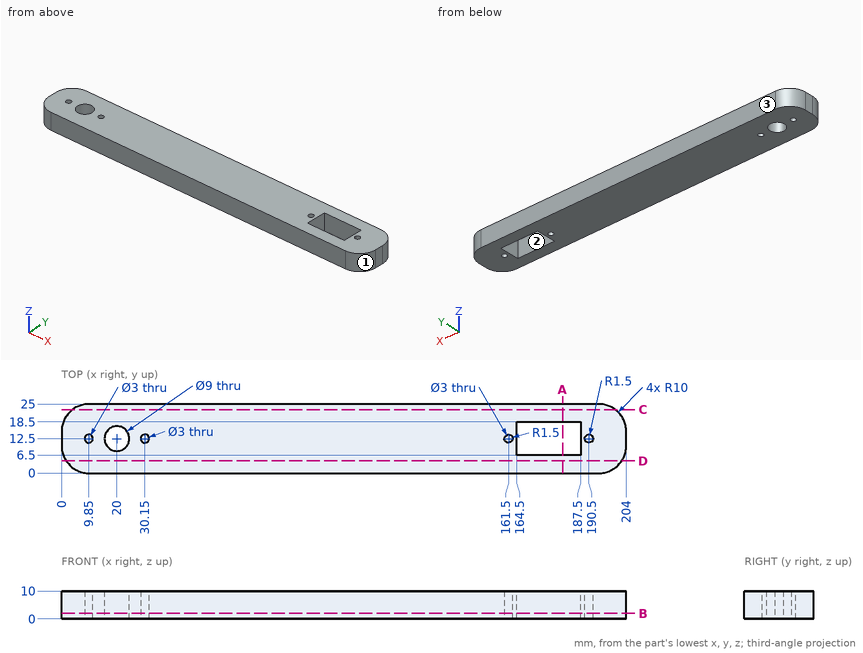
Can you work these out from the drawing? Everything is in mm from the part's minimum corner. Round coordinates to 2 decimals unless told otherwise and drop trailing zeros. Loops run counter-clockwise (first coordinate to the right, second up) from the corner with the lowest first, then second, coordinate; pieces in that order, holes last. Notation, with made-up numbers: (70.25, 79.5) - (124.25, 79.5) arc R26 cw to (124.25, 93.5) - close; hole circle Ø3 at (-11.5, 26.25). An arc over 180 degrees is marked (long way). Answer in a Markdown table with one row per item. Add a question column.
Q1. We'd pull the mould along X, two halves only. Please class the marked faces 1, 2 and 3: pulls with the +X half, pulls with the -X half, needs draft (parallel to the pull), parting line crosses it, or undercut.
Q2. I need wall thicknesses on L1, parallel to Y at x = 179, z = 4.5; L2, parallel to X at y = 9, z = 4; L3, parallel to X at y = 10.5, z = 4.5. Which ranges of each line are inside material? Lowest first, please.
Q3. For pin 1 Ø4 at (y, z) = (12, 6) entering from -X, with a flat end and sliding along its axis, tell me the tip position at first contact or that it passes through.
Q4. I want a section at C-C on y = 23. List the corners of the cut face in (x, z) for me.
Q5. I want a section at B-B on z = 2. List the corners of the cut face in (x, y) for me, and give its area (3 significant figures).
Q6. I want a section at D-D on y = 4.5. List the corners of the cut face in (x, z) for me.
Q7. I want a section at A-A on x = 181. List the corners of the cut face in (y, z) for me.
A:
| question | item | result |
|---|---|---|
| 1 | face 1 | pulls with the +X half |
| 1 | face 2 | undercut |
| 1 | face 3 | needs draft |
| 2 | L1 | 0 to 6.5, 18.5 to 25 |
| 2 | L2 | 0.05 to 17.17, 22.83 to 164.5, 187.5 to 203.95 |
| 2 | L3 | 0 to 15.97, 24.03 to 164.5, 187.5 to 204 |
| 3 | pin 1 | x = 0 |
| 4 | outline | (4, 0) - (200, 0) - (200, 10) - (4, 10) - close |
| 5 | outline | (0, 10) arc R10 ccw to (10, 0) - (194, 0) arc R10 ccw to (204, 10) - (204, 15) arc R10 ccw to (194, 25) - (10, 25) arc R10 ccw to (0, 15) - close; hole circle Ø3 at (9.85, 12.5); hole circle Ø9 at (20, 12.5); hole circle Ø3 at (30.15, 12.5); hole circle Ø3 at (161.5, 12.5); hole (164.5, 6.5) - (187.5, 6.5) - (187.5, 18.5) - (164.5, 18.5) - close; hole circle Ø3 at (190.5, 12.5) |
| 5 | area | 4,650 mm^2 |
| 6 | outline | (1.65, 0) - (202.35, 0) - (202.35, 10) - (1.65, 10) - close |
| 7 | outline | (0, 0) - (6.5, 0) - (6.5, 10) - (0, 10) - close; (18.5, 0) - (25, 0) - (25, 10) - (18.5, 10) - close |
